from build123d import *

# Parameters (mm, degrees)
SKETCH1_R           = 2.4
BOSS_EXTRUDE1_DEPTH = 1.6
CUT_EXTRUDE1_REACH  = 232.538
SKETCH2_W           = 10
SKETCH2_H           = 33
FILLET1_R           = 3


with BuildPart() as part:
    # Sketch1 → Boss-Extrude1 (new body)
    with BuildSketch(Plane(origin=(0, 0, 0), x_dir=(1, 0, 0), z_dir=(0, 1, 0))):
        Polygon((0, 132), (189, 132), (189, 0), (0, 0), (-10, 0), (-10, 132), align=None)
        with Locations(Location((6, 96, 0), (0, 0, 270))):
            Circle(SKETCH1_R, mode=Mode.SUBTRACT)
        with Locations(Location((6, 36, 0), (0, 0, 270))):
            Circle(SKETCH1_R, mode=Mode.SUBTRACT)
        with Locations(Location((183, 66, 0), (0, 0, 270))):
            Circle(SKETCH1_R, mode=Mode.SUBTRACT)
    extrude(amount=BOSS_EXTRUDE1_DEPTH)

    # Sketch2 → Cut-Extrude1 (cut, up to next)
    with BuildSketch(Plane(origin=(0, 1.6, 0), x_dir=(1, 0, 0), z_dir=(0, 1, 0)), mode=Mode.PRIVATE) as cut_extrude1_sk1:
        with Locations((-5, 115.5)):
            Rectangle(SKETCH2_W, SKETCH2_H)
    cut_extrude1_tool1 = extrude(cut_extrude1_sk1.sketch, amount=-CUT_EXTRUDE1_REACH, mode=Mode.PRIVATE) & part.part
    cut_extrude1 = cut_extrude1_tool1.solids().sort_by_distance((-5, 1.6, -115.5))[0]
    add(cut_extrude1, mode=Mode.SUBTRACT)

    # Mirror1: Cut-Extrude1 across plane
    add(cut_extrude1.mirror(Plane.XY.offset(-66)), mode=Mode.SUBTRACT)

    # Fillet1
    fillet1_edges = [part.edges().sort_by_distance(p)[0] for p in [
        (189, 0.8, -132),
        (189, 0.8, 0),
        (-10, 0.8, -99),
        (0, 0.8, -132),
        (-10, 0.8, -33),
        (0, 0.8, 0),
    ]]
    fillet(fillet1_edges, radius=FILLET1_R)


solid = part.part
CAD build for the part. Positions are in the model's coordinates, mm. Coordinates: 2 decimals unless noted, no trailing zeros. Write each loop counter-clockwise with the first axis right and the second up, starting at its lowest first coordinate (ties: lowest second). Pieces come first, ordered by that corner, then holes. Notation, with made-up numbers: M 79.5,88 L 92.5,88 A16 ccw 92.5,115 Z; hole C 79.25,36 d7. An arc over 180 degrees is marked long. Return JSON: item names as keys, results as strings.
Item 1: Slice it at B-B, the plane x = 6. Write the cut outline in (y, z).
Findings below:
{"outline": "M 0,-132 L 1.6,-132 L 1.6,-98.4 L 0,-98.4 Z; M 0,-93.6 L 1.6,-93.6 L 1.6,-38.4 L 0,-38.4 Z; M 0,-33.6 L 1.6,-33.6 L 1.6,0 L 0,0 Z"}
Item 2: Probe line 1 (X direction, y = 1.1, z = -66); line 2 (X direction, y = 0.45, z = -96); line 3 (X direction, y = 0.7, z = -112). List the from-to ranges inside material, lowest first. Write a range as from..to.
Findings below:
{"line 1": "x = -10..180.6, 185.4..189", "line 2": "x = -10..3.6, 8.4..189", "line 3": "x = 0..189"}
Item 3: Drop a flat-ended pin along its axis: pin 1 Ø0.5 at (x, y) = (-5, 0.5) entering from -Z. Give the stop position or say it passes through.
Findings below:
{"pin 1": "stops at z = -99"}
Item 4: Two-plate mould, pull along Z, no slides. Class faces 1 (the flat face through (91, 1.6, -67)), 2 (the cylindrical face through (6.106, 0.789, -38.398)): +Z half, -Z half, draft (parallel to the pull), parting line (faces both ways), or undercut.
Findings below:
{"face 1": "draft", "face 2": "undercut"}
Item 5: Slice it at D-D, the plane z = -109.5. Write the cut outline in (x, y), and give its area (3 significant figures).
Findings below:
{"outline": "M 0,0 L 189,0 L 189,1.6 L 0,1.6 Z", "area": "302 mm2"}
Item 6: Slice it at C-C, the plane z = -66. Write the cut outline in (x, y), and give its area (3 significant figures).
Findings below:
{"outline": "M -10,0 L 180.6,0 L 180.6,1.6 L -10,1.6 Z; M 185.4,0 L 189,0 L 189,1.6 L 185.4,1.6 Z", "area": "311 mm2"}
Item 7: Slice it at A-A, the plane y = 1.25. Write the cut outline in (x, z), and give its area (3 significant figures).
Findings below:
{"outline": "M -10,-96 A3 ccw -7,-99 L 0,-99 L 0,-129 A3 ccw 3,-132 L 186,-132 A3 ccw 189,-129 L 189,-3 A3 ccw 186,0 L 3,0 A3 ccw 0,-3 L 0,-33 L -7,-33 A3 ccw -10,-36 Z; hole C 6,-96 d4.8; hole C 6,-36 d4.8; hole C 183,-66 d4.8", "area": "25,500 mm2"}
